```python
from build123d import *

# Parameters (mm, degrees)
F0_R     = 4.78
F1_DEPTH = 3


with BuildPart() as f1:
    # F0 (on Top) → F1 (new body)
    with BuildSketch(Plane.XY):
        with Locations((0, -1.897358)):
            Circle(F0_R)
        with BuildLine():
            Line((-1.5, -3.651894), (-1.5, -0.151894))
            ThreePointArc((-1.5, -0.151894), (0, 0.390902), (1.5, -0.151894))
            Line((1.5, -0.151894), (1.5, -3.651894))
            ThreePointArc((1.5, -3.651894), (0, -4.19469), (-1.5, -3.651894))
        make_face(mode=Mode.SUBTRACT)
    extrude(amount=F1_DEPTH)


solid = f1.part
```
Can you work these out from the model? Positions are in its coordinate system, mm. A direction names the side the tool comes from. Coordinates: 2 decimals unless noted, no trailing zeros. Loops run counter-clockwise (first coordinate to the right, second up) from the corner with the lowest first, then second, coordinate; pieces in that order, holes last.
1) Thinking about a two-plate mould opening in Y: for faces 3 (the cylindrical face through (4.56, -0.46, 1.48)), 4 (the flat face through (2, -2, 0)), 5 (the cylindrical face through (0.023, -4.195, 1.479)), which applies, pulls with the +Y half, pulls with the -Y half, needs draft (parallel to the pull), parting line crosses it, or undercut?
2) Which directions (+Z, -Z, +X, -X, +Y, -Y) give clear straight access to the entire face, cutting with the end or side of a thin tool? Please do faces 1 (the cylindrical face through (-0.02, 0.39, 1.48)), 2 (the flat face through (2, -2, 3)).
3) For pin 1 (1 mm diameter, centred on x = -2.5, z = 2.5, fed in from +Y), with a flat end and sliding along its axis, tell me the tip position at first contact or that it passes through.
4) I need wall thicknesses on probe 1 along Y at (x, z) = (0, 2.8); probe 2 along Y at (x, z) = (1.25, 1.3); probe 3 along X at (y, z) = (-0.5, 1.6). Which ranges of each line are inside material? Lowest first, please.
5) Imagine slicing it at C-C on z = 0.65. List the corners of the cut face in (x, y) for me.
6) Imagine slicing it at B-B on y = -3. List the corners of the cut face in (x, z) for me, plus the area to 3 significant figures.
7) Imagine slicing it at A-A on x = 0. List the corners of the cut face in (y, z) for me.
8) Imagine slicing it at D-D on x = 4. List the corners of the cut face in (y, z) for me.
Completed:
1. face 3: parting line crosses it
1. face 4: needs draft
1. face 5: undercut
2. face 1: +Z, -Z
2. face 2: +Z, +X, -X, +Y, -Y
3. pin 1: stops at y = 2.44
4. probe 1: y = -6.68 to -4.19, 0.39 to 2.88
4. probe 2: y = -6.51 to -3.83, 0.03 to 2.72
4. probe 3: x = -4.57 to -1.5, 1.5 to 4.57
5. outline: circle Ø9.56 at (0, -1.9); hole (-1.5, -3.65) arc R2.34 ccw to (1.5, -3.65) - (1.5, -0.15) arc R2.34 ccw to (-1.5, -0.15) - close
6. outline: (-4.65, 0) - (-1.5, 0) - (-1.5, 3) - (-4.65, 3) - close; (1.5, 0) - (4.65, 0) - (4.65, 3) - (1.5, 3) - close
6. area: 18.9 mm2
7. outline: (-6.68, 0) - (-4.19, 0) - (-4.19, 3) - (-6.68, 3) - close; (0.39, 0) - (2.88, 0) - (2.88, 3) - (0.39, 3) - close
8. outline: (-4.51, 0) - (0.72, 0) - (0.72, 3) - (-4.51, 3) - close
